from build123d import *

# Parameters (mm, degrees)
SKETCH_2_R               = 1.75
EXTRUDE_937_DEPTH        = 5
FILLET_1_R               = 1
SKETCH_9_W               = 3
SKETCH_9_H               = 7.5
CUT_EXTRUDE_1306_DEPTH   = 8
CUT_EXTRUDE_2_DEPTH      = 10
CUT_EXTRUDE_2_DEPTH_BACK = 5
SKETCH_12_R              = 2.2
CUT_EXTRUDE_START        = -10
SKETCH_15_R              = 10.175
SKETCH_15_R_2            = 9.8
CUT_EXTRUDE_1_DEPTH      = 10
SKETCH_16_R              = 2.2
CUT_EXTRUDE_1_2_DEPTH    = 41.324759764
SKETCH_18_R              = 10.175
SKETCH_18_R_2            = 9.988159657
CUT_EXTRUDE_2_2_DEPTH    = 3.5


with BuildPart() as part:
    # Эскиз1 → Revolve 727 (revolve)
    with BuildSketch(Plane(origin=(0, 0, 0), x_dir=(0, 0, -1), z_dir=(1, 0, 0)), mode=Mode.PRIVATE) as revolve_727_sk:
        Polygon((0, 0), (0, 7.025), (16.5, 7.025), (16.5, 8.025), (21, 8.025), (21, 7.025), (31, 7.025), (31, -1.4), (14.5, -1.4), (14.5, 0), align=None)
    revolve(revolve_727_sk.sketch.rotate(Axis((0, -3.15, 0), (0, 0, -1)), 90), axis=Axis((0, -3.15, 0), (0, 0, -1)))

    # Эскиз2 → Extrude 937 (add)
    with BuildSketch(Plane(origin=(0, 0, -31), x_dir=(-1, 0, 0), z_dir=(0, 0, -1))):
        Polygon((4.994079828, 5.5), (-4.994079828, 5.5), (-9.988159657, -3.15), (-4.994079828, -11.8), (4.994079828, -11.8), (9.988159657, -3.15), align=None)
        with Locations(Location((0, -3.15, 0), (0, 0, 180))):
            Circle(SKETCH_2_R, mode=Mode.SUBTRACT)
    extrude(amount=EXTRUDE_937_DEPTH)

    # Скругление1
    fillet_1_edges = [part.edges().sort_by_distance(p)[0] for p in [
        (-3.15, -3.15, -14.5),
    ]]
    fillet(fillet_1_edges, radius=FILLET_1_R)

    # Эскиз9 → Cut-Extrude 1306 (cut)
    with BuildSketch(Plane.XY):
        with Locations((5.5, -3.15)):
            Rectangle(SKETCH_9_W, SKETCH_9_H)
        Polygon((-6.747595264, -7.337177826), (-5.247595264, -4.739101615), (1.247595264, -8.489101615), (-0.252404736, -11.087177826), align=None)
    extrude(amount=-CUT_EXTRUDE_1306_DEPTH, mode=Mode.SUBTRACT)

    # Эскиз12 → Cut-Extrude 2 (cut, two sides: drawn at the far end of the back side and taken through both)
    with BuildSketch(Plane(origin=(-3.363990011, -5.826601615, 0), x_dir=(0.8660254037844364, -0.500000000000004, 0), z_dir=(-0.500000000000004, -0.8660254037844365, 0)).offset(-CUT_EXTRUDE_2_DEPTH_BACK)):
        with Locations(Location((1.575, -3.5, 0), (0, 0, 180))):
            Circle(SKETCH_12_R)
    extrude(amount=CUT_EXTRUDE_2_DEPTH + CUT_EXTRUDE_2_DEPTH_BACK, mode=Mode.SUBTRACT)

    # Эскиз15 → Cut-Extrude 1 (cut)
    with BuildSketch(Plane.XY.offset(CUT_EXTRUDE_START)):
        with Locations((0, -3.15)):
            Circle(SKETCH_15_R)
        with Locations((0, -3.15)):
            Circle(SKETCH_15_R_2, mode=Mode.SUBTRACT)
    extrude(amount=CUT_EXTRUDE_1_DEPTH, mode=Mode.SUBTRACT)

    # Эскиз16 → Cut-Extrude 1 2 (cut, through all)
    with BuildSketch(Plane(origin=(0, 0, 0), x_dir=(0, 0, -1), z_dir=(1, 0, 0))):
        with Locations(Location((3.5, -3.15, 0), (0, 0, 180))):
            Circle(SKETCH_16_R)
    extrude(amount=CUT_EXTRUDE_1_2_DEPTH, mode=Mode.SUBTRACT)

    # Эскиз18 → Cut-Extrude 2 2 (cut)
    with BuildSketch(Plane(origin=(0, 0, -31), x_dir=(-1, 0, 0), z_dir=(0, 0, -1))):
        with Locations(Location((0, -3.15, 0), (0, 0, 180))):
            Circle(SKETCH_18_R)
        with Locations((0, -3.15)):
            Circle(SKETCH_18_R_2, mode=Mode.SUBTRACT)
    extrude(amount=-CUT_EXTRUDE_2_2_DEPTH, mode=Mode.SUBTRACT)


solid = part.part
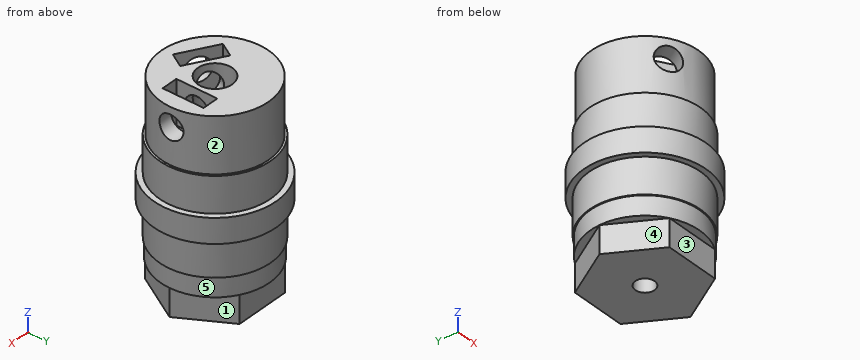
For this review, take the finished solid that the model builds, in its own axes (mm). Face numbers are marked on the shaded views. A direction names the side the tool comes from. Give positions to 0.01 mm unless a question says otherwise; leave off trailing zeros. Write each loop counter-clockwise with the first axis right and the second up, starting at its lowest first coordinate (ties: lowest second). Pieces come first, ordered by that corner, then holes. Notation, with made-up numbers: (-7, 43.5) -> (33, 43.5) arc R18 cw to (33, 70.5) -> close; hole circle Ø4 at (84.5, -2.75). An arc over 180 degrees is marked (long way). Use CSV: the item, a comma, the result in double quotes.
Q1. To check wall thickness, follow probe 1 along X at (y, z) = (-6, -4); probe 2 along Y at (x, z) = (0, -30.25); probe 3 along Y at (x, z) = (2.5, -32). State the ranges of each line that lie inside material, in increasing order. Write a range as [from, to].
Conclusion:
probe 1,"[-9.38, -5.98], [1.34, 4], [7, 9.38]"
probe 2,"[-13.14, -4.9], [-1.4, 6.84]"
probe 3,"[-11.8, 5.5]"
Q2. For P1, Ø2, axis at y = -11, z = -11.5, coming from the +X side; P2, Ø5, axis at y = 1.5, z = -13, coming from the +X side; P3, Ø0.7, axis at x = -1.5, y = -12.5, coming from the -Z side, all flat-tipped, find the tip position at first contact; note any pin that passes through.
Conclusion:
P1,"x = 7.52"
P2,"x = 9.95"
P3,"z = -31"
Q3. Take a section at D-D, the plane y = 6. Write out the cut boundary in (x, z).
Conclusion:
outline,"(-6.42, -21) -> (-4.45, -21) -> (-4.45, -27.5) -> (-4.01, -27.5) -> (-4.01, -31) -> (4.01, -31) -> (4.01, -27.5) -> (4.45, -27.5) -> (4.45, -21) -> (6.42, -21) -> (6.42, -16.5) -> (4.45, -16.5) -> (4.45, -10) -> (3.51, -10) -> (3.51, 0) -> (-3.51, 0) -> (-3.51, -10) -> (-4.45, -10) -> (-4.45, -16.5) -> (-6.42, -16.5) -> close"
Q4. Tool access review of the marked faces 1, 2, 3, 4 and 5: name each direction out of +Z, -Z, +X, -X, +Y, -Y from which nothing blocks a thin tool from reaching the whole face with its end or side.
Conclusion:
face 1,"-Z, +X, +Y"
face 2,"+Z"
face 3,"-Z, +X, -X, -Y"
face 4,"-Z, -X, -Y"
face 5,"-Z"
Q5. Take a section at C-C, the plane z = -10.5. Write out the cut boundary in (x, y) (3 decimals).
Conclusion:
outline,"circle Ø20.35 at (0, -3.15); hole circle Ø6.3 at (0, -3.15)"
Q6. Take a section at A-A, the plane x = 8. Write out the cut boundary in (y, z), then the cut area to 3 significant figures.
Conclusion:
outline,"(-10.95, -21) -> (-9.44, -21) -> (-9.44, -27.5) -> (-9.13, -27.5) -> (-9.13, -31) -> (-6.59, -31) -> (-6.59, -36) -> (0.29, -36) -> (0.29, -31) -> (2.83, -31) -> (2.83, -27.5) -> (3.14, -27.5) -> (3.14, -21) -> (4.65, -21) -> (4.65, -16.5) -> (3.14, -16.5) -> (3.14, -10) -> (2.51, -10) -> (2.51, 0) -> (-8.81, 0) -> (-8.81, -10) -> (-9.44, -10) -> (-9.44, -16.5) -> (-10.95, -16.5) -> close; hole circle Ø4.4 at (-3.15, -3.5)"
area,"408 mm2"
Q7. Take a section at B-B, the plane y = 2.5. Write out the cut boundary in (x, z).
Conclusion:
outline,"(-9.64, -21) -> (-8.46, -21) -> (-8.46, -27.5) -> (-8.24, -27.5) -> (-8.24, -31) -> (-6.73, -31) -> (-6.73, -36) -> (6.73, -36) -> (6.73, -31) -> (8.24, -31) -> (8.24, -27.5) -> (8.46, -27.5) -> (8.46, -21) -> (9.64, -21) -> (9.64, -16.5) -> (8.46, -16.5) -> (8.46, -10) -> (8.01, -10) -> (8.01, 0) -> (-8.01, 0) -> (-8.01, -10) -> (-8.46, -10) -> (-8.46, -16.5) -> (-9.64, -16.5) -> close"
